Can you work these out from the model? Positions are in its coordinate system, mm. Give positions to 0.01 mm unless a question says otherwise; leave off trailing zeros. Loops run counter-clockwise (first coordinate to the right, second up) from the corner with the lowest first, then second, coordinate; pieces in that order, holes last. Notation, with made-up numbers: M 61,6.25 L 93,6.25 A21 cw 93,10.25 Z; hole C -16.5,-29.75 d4. An arc over 180 degrees is marked long. Use CSV: the item, a comma, the result in double quotes.
from build123d import *

# Parameters (mm, degrees)
F0_R     = 14.2875
F0_R_2   = 2.54
F0_R_3   = 3.175
F0_R_4   = 8.89
F1_DEPTH = 6.35
F2_R     = 6.35


with BuildPart() as f1:
    # F0 (on Right) → F1 (new body)
    with BuildSketch(Plane.YZ):
        Polygon((0, 406.4), (0, 0), (101.6, 0), (101.6, 152.4), (101.6, 190.5), (101.6, 406.4), align=None)
        with BuildLine():
            ThreePointArc((14.868026, 8.518026), (13.483992, 8.242724), (12.7, 9.416051))
            Line((12.7, 9.416051), (12.7, 36.83))
            ThreePointArc((12.7, 36.83), (13.071974, 37.728026), (13.97, 38.1))
            Line((13.97, 38.1), (41.383949, 38.1))
            ThreePointArc((41.383949, 38.1), (42.557276, 37.316008), (42.281974, 35.931974))
            Line((42.281974, 35.931974), (14.868026, 8.518026))
        make_face(mode=Mode.SUBTRACT)
        with BuildLine():
            Line((41.383949, 50.8), (13.97, 50.8))
            ThreePointArc((13.97, 50.8), (13.071974, 51.171974), (12.7, 52.07))
            Line((12.7, 52.07), (12.7, 79.483949))
            ThreePointArc((12.7, 79.483949), (13.483992, 80.657276), (14.868026, 80.381974))
            Line((14.868026, 80.381974), (42.281974, 52.968026))
            ThreePointArc((42.281974, 52.968026), (42.557276, 51.583992), (41.383949, 50.8))
        make_face(mode=Mode.SUBTRACT)
        with BuildLine():
            Line((88.9, 36.83), (88.9, 9.416051))
            ThreePointArc((88.9, 9.416051), (88.116008, 8.242724), (86.731974, 8.518026))
            Line((86.731974, 8.518026), (59.318026, 35.931974))
            ThreePointArc((59.318026, 35.931974), (59.042724, 37.316008), (60.216051, 38.1))
            Line((60.216051, 38.1), (87.63, 38.1))
            ThreePointArc((87.63, 38.1), (88.528026, 37.728026), (88.9, 36.83))
        make_face(mode=Mode.SUBTRACT)
        with BuildLine():
            ThreePointArc((60.216051, 50.8), (59.042724, 51.583992), (59.318026, 52.968026))
            Line((59.318026, 52.968026), (86.731974, 80.381974))
            ThreePointArc((86.731974, 80.381974), (88.116008, 80.657276), (88.9, 79.483949))
            Line((88.9, 79.483949), (88.9, 52.07))
            ThreePointArc((88.9, 52.07), (88.528026, 51.171974), (87.63, 50.8))
            Line((87.63, 50.8), (60.216051, 50.8))
        make_face(mode=Mode.SUBTRACT)
        with BuildLine():
            ThreePointArc((14.868026, 97.418026), (13.483992, 97.142724), (12.7, 98.316051))
            Line((12.7, 98.316051), (12.7, 125.73))
            ThreePointArc((12.7, 125.73), (13.071974, 126.628026), (13.97, 127))
            Line((13.97, 127), (41.383949, 127))
            ThreePointArc((41.383949, 127), (42.557276, 126.216008), (42.281974, 124.831974))
            Line((42.281974, 124.831974), (14.868026, 97.418026))
        make_face(mode=Mode.SUBTRACT)
        with BuildLine():
            Line((41.383949, 139.7), (13.97, 139.7))
            ThreePointArc((13.97, 139.7), (13.071974, 140.071974), (12.7, 140.97))
            Line((12.7, 140.97), (12.7, 168.383949))
            ThreePointArc((12.7, 168.383949), (13.483992, 169.557276), (14.868026, 169.281974))
            Line((14.868026, 169.281974), (42.281974, 141.868026))
            ThreePointArc((42.281974, 141.868026), (42.557276, 140.483992), (41.383949, 139.7))
        make_face(mode=Mode.SUBTRACT)
        with BuildLine():
            ThreePointArc((14.868026, 186.318026), (13.483992, 186.042724), (12.7, 187.216051))
            Line((12.7, 187.216051), (12.7, 214.63))
            ThreePointArc((12.7, 214.63), (13.071974, 215.528026), (13.97, 215.9))
            Line((13.97, 215.9), (41.383949, 215.9))
            ThreePointArc((41.383949, 215.9), (42.557276, 215.116008), (42.281974, 213.731974))
            Line((42.281974, 213.731974), (14.868026, 186.318026))
        make_face(mode=Mode.SUBTRACT)
        with BuildLine():
            Line((88.9, 125.73), (88.9, 98.316051))
            ThreePointArc((88.9, 98.316051), (88.116008, 97.142724), (86.731974, 97.418026))
            Line((86.731974, 97.418026), (59.318026, 124.831974))
            ThreePointArc((59.318026, 124.831974), (59.042724, 126.216008), (60.216051, 127))
            Line((60.216051, 127), (87.63, 127))
            ThreePointArc((87.63, 127), (88.528026, 126.628026), (88.9, 125.73))
        make_face(mode=Mode.SUBTRACT)
        with BuildLine():
            ThreePointArc((60.216051, 139.7), (59.042724, 140.483992), (59.318026, 141.868026))
            Line((59.318026, 141.868026), (86.731974, 169.281974))
            ThreePointArc((86.731974, 169.281974), (88.116008, 169.557276), (88.9, 168.383949))
            Line((88.9, 168.383949), (88.9, 140.97))
            ThreePointArc((88.9, 140.97), (88.528026, 140.071974), (87.63, 139.7))
            Line((87.63, 139.7), (60.216051, 139.7))
        make_face(mode=Mode.SUBTRACT)
        with BuildLine():
            Line((88.9, 214.63), (88.9, 187.216051))
            ThreePointArc((88.9, 187.216051), (88.116008, 186.042724), (86.731974, 186.318026))
            Line((86.731974, 186.318026), (59.318026, 213.731974))
            ThreePointArc((59.318026, 213.731974), (59.042724, 215.116008), (60.216051, 215.9))
            Line((60.216051, 215.9), (87.63, 215.9))
            ThreePointArc((87.63, 215.9), (88.528026, 215.528026), (88.9, 214.63))
        make_face(mode=Mode.SUBTRACT)
        with BuildLine():
            Line((41.383949, 228.6), (13.97, 228.6))
            ThreePointArc((13.97, 228.6), (13.071974, 228.971974), (12.7, 229.87))
            Line((12.7, 229.87), (12.7, 257.283949))
            ThreePointArc((12.7, 257.283949), (13.483992, 258.457276), (14.868026, 258.181974))
            Line((14.868026, 258.181974), (42.281974, 230.768026))
            ThreePointArc((42.281974, 230.768026), (42.557276, 229.383992), (41.383949, 228.6))
        make_face(mode=Mode.SUBTRACT)
        with BuildLine():
            ThreePointArc((14.868026, 275.218026), (13.483992, 274.942724), (12.7, 276.116051))
            Line((12.7, 276.116051), (12.7, 303.53))
            ThreePointArc((12.7, 303.53), (13.071974, 304.428026), (13.97, 304.8))
            Line((13.97, 304.8), (41.383949, 304.8))
            ThreePointArc((41.383949, 304.8), (42.557276, 304.016008), (42.281974, 302.631974))
            Line((42.281974, 302.631974), (14.868026, 275.218026))
        make_face(mode=Mode.SUBTRACT)
        with BuildLine():
            ThreePointArc((60.216051, 228.6), (59.042724, 229.383992), (59.318026, 230.768026))
            Line((59.318026, 230.768026), (86.731974, 258.181974))
            ThreePointArc((86.731974, 258.181974), (88.116008, 258.457276), (88.9, 257.283949))
            Line((88.9, 257.283949), (88.9, 229.87))
            ThreePointArc((88.9, 229.87), (88.528026, 228.971974), (87.63, 228.6))
            Line((87.63, 228.6), (60.216051, 228.6))
        make_face(mode=Mode.SUBTRACT)
        with BuildLine():
            Line((88.9, 303.53), (88.9, 276.116051))
            ThreePointArc((88.9, 276.116051), (88.116008, 274.942724), (86.731974, 275.218026))
            Line((86.731974, 275.218026), (59.318026, 302.631974))
            ThreePointArc((59.318026, 302.631974), (59.042724, 304.016008), (60.216051, 304.8))
            Line((60.216051, 304.8), (87.63, 304.8))
            ThreePointArc((87.63, 304.8), (88.528026, 304.428026), (88.9, 303.53))
        make_face(mode=Mode.SUBTRACT)
        with BuildLine():
            ThreePointArc((13.97, 317.5), (13.071974, 317.871974), (12.7, 318.77))
            Line((12.7, 318.77), (12.7, 346.183949))
            ThreePointArc((12.7, 346.183949), (13.483992, 347.357276), (14.868026, 347.081974))
            Line((14.868026, 347.081974), (42.281974, 319.668026))
            ThreePointArc((42.281974, 319.668026), (42.557276, 318.283992), (41.383949, 317.5))
            Line((41.383949, 317.5), (13.97, 317.5))
        make_face(mode=Mode.SUBTRACT)
        with BuildLine():
            Line((12.7, 365.016051), (12.7, 392.43))
            ThreePointArc((12.7, 392.43), (13.071974, 393.328026), (13.97, 393.7))
            Line((13.97, 393.7), (41.383949, 393.7))
            ThreePointArc((41.383949, 393.7), (42.557276, 392.916008), (42.281974, 391.531974))
            Line((42.281974, 391.531974), (14.868026, 364.118026))
            ThreePointArc((14.868026, 364.118026), (13.483992, 363.842724), (12.7, 365.016051))
        make_face(mode=Mode.SUBTRACT)
        with BuildLine():
            Line((87.63, 317.5), (60.216051, 317.5))
            ThreePointArc((60.216051, 317.5), (59.042724, 318.283992), (59.318026, 319.668026))
            Line((59.318026, 319.668026), (86.731974, 347.081974))
            ThreePointArc((86.731974, 347.081974), (88.116008, 347.357276), (88.9, 346.183949))
            Line((88.9, 346.183949), (88.9, 318.77))
            ThreePointArc((88.9, 318.77), (88.528026, 317.871974), (87.63, 317.5))
        make_face(mode=Mode.SUBTRACT)
        with BuildLine():
            Line((60.216051, 393.7), (87.63, 393.7))
            ThreePointArc((87.63, 393.7), (88.528026, 393.328026), (88.9, 392.43))
            Line((88.9, 392.43), (88.9, 365.016051))
            ThreePointArc((88.9, 365.016051), (88.116008, 363.842724), (86.731974, 364.118026))
            Line((86.731974, 364.118026), (59.318026, 391.531974))
            ThreePointArc((59.318026, 391.531974), (59.042724, 392.916008), (60.216051, 393.7))
        make_face(mode=Mode.SUBTRACT)
        Polygon((101.6, 152.4), (101.6, 0), (228.6, 0), (228.6, 152.4), (139.7, 152.4), align=None)
        with Locations((146.05, 50.8)):
            Circle(F0_R, mode=Mode.SUBTRACT)
        with Locations((168.275, 98.425)):
            Circle(F0_R_2, mode=Mode.SUBTRACT)
        with Locations((215.9, 12.7)):
            Circle(F0_R_3, mode=Mode.SUBTRACT)
        with Locations((200.025, 98.425)):
            Circle(F0_R_2, mode=Mode.SUBTRACT)
        with Locations((152.4, 139.7)):
            Circle(F0_R_3, mode=Mode.SUBTRACT)
        with Locations((168.275, 130.175)):
            Circle(F0_R_2, mode=Mode.SUBTRACT)
        with Locations((184.15, 114.3)):
            Circle(F0_R_4, mode=Mode.SUBTRACT)
        with Locations((200.025, 130.175)):
            Circle(F0_R_2, mode=Mode.SUBTRACT)
        with Locations((215.9, 139.7)):
            Circle(F0_R_3, mode=Mode.SUBTRACT)
        with BuildLine():
            Line((101.6, 190.5), (101.6, 152.4))
            Line((101.6, 152.4), (139.7, 152.4))
            ThreePointArc((139.7, 152.4), (112.759232, 163.559232), (101.6, 190.5))
        make_face()
    extrude(amount=F1_DEPTH)

    # F2
    f2_edges = [f1.edges().sort_by_distance(p)[0] for p in [
        (3.175, 228.6, 0),
        (3.175, 228.6, 152.4),
        (3.175, 0, 0),
        (3.175, 0, 406.4),
        (3.175, 101.6, 406.4),
    ]]
    fillet(f2_edges, radius=F2_R)


solid = f1.part
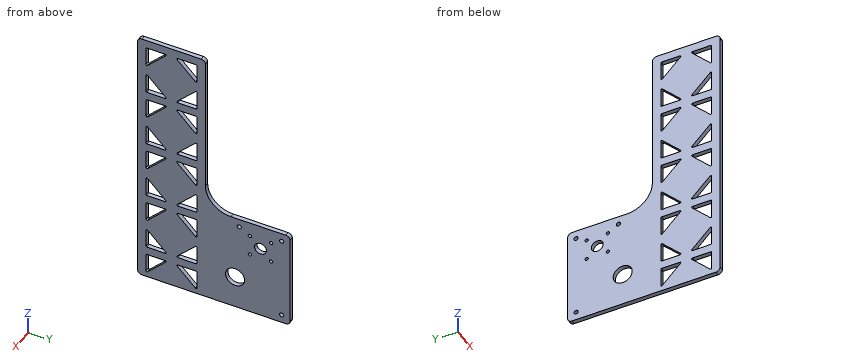
Q1. I'm going to push flat-ended pins straight in: P1, Ø6, axis at y = 168.275, z = 98.425, coming from the -X side; P2, Ø1, axis at x = 5.5, y = 128, coming from the +Z side; P3, Ø3, axis at x = 2, z = 205.5, coming from the +Y side. Where does each tip first touch, or does it pass through?
Model answer:
P1,"x = 0"
P2,"z = 154.41"
P3,"y = 101.6"
Q2. Please list where these lines run through material, in increasing order: L1, parallel to Z at x = 3.75, y = 215.9 (3 decimals); L2, parallel to Z at x = 4.75, y = 184.15; L3, parallel to Y at x = 3.5, z = 57.5. Write a range as from..to.
Model answer:
L1,"0..9.525, 15.875..136.525, 142.875..152.4"
L2,"0..105.41, 123.19..152.4"
L3,"0..12.7, 37.75..63.85, 88.9..133.43, 158.67..228.6"
Q3. I want a section at D-D, the plane z = 289.5. Please give me the cut outline in (x, y), then the cut area to 3 significant figures.
Model answer:
outline,"M 0,0 L 6.35,0 L 6.35,12.7 L 0,12.7 Z; M 0,29.15 L 6.35,29.15 L 6.35,72.45 L 0,72.45 Z; M 0,88.9 L 6.35,88.9 L 6.35,101.6 L 0,101.6 Z"
area,"436 mm2"
Q4. I want a section at C-C, the plane y = 189. Please give me the cut outline in (x, z).
Model answer:
outline,"M 0,0 L 6.35,0 L 6.35,106.85 L 0,106.85 Z; M 0,121.75 L 6.35,121.75 L 6.35,152.4 L 0,152.4 Z"
Q5. I want a section at B-B, the plane z = 372. Please give me the cut outline in (x, y).
Model answer:
outline,"M 0,0 L 6.35,0 L 6.35,12.7 L 0,12.7 Z; M 0,22.75 L 6.35,22.75 L 6.35,78.85 L 0,78.85 Z; M 0,88.9 L 6.35,88.9 L 6.35,101.6 L 0,101.6 Z"
Q6. I want a section at A-A, the plane z = 114.3. Please give me the cut outline in (x, y).
Model answer:
outline,"M 0,0 L 6.35,0 L 6.35,12.7 L 0,12.7 Z; M 0,31.75 L 6.35,31.75 L 6.35,69.85 L 0,69.85 Z; M 0,88.9 L 6.35,88.9 L 6.35,175.26 L 0,175.26 Z; M 0,193.04 L 6.35,193.04 L 6.35,228.6 L 0,228.6 Z"
